Autodesk Inventor part; units mm, degrees
ref_plane "YZ Plane" through (0, 0, 0) normal (1, 0, 0) x (0, 1, 0)
ref_plane "XZ Plane" through (0, 0, 0) normal (0, 1, 0) x (-1, 0, 0)
ref_plane "XY Plane" through (0, 0, 0) normal (0, 0, 1) x (1, 0, 0)
sketch "Sketch5" plane through (0, 0, 0) normal (0, 0, 1) x (1, 0, 0)
  line L0 (27.5, -18) -> (0, -18)
  line L1 (0, -18) -> (0, 0)
  line L2 (27.5, -1.0645) -> (27.5, -18)
  line L3 (1.6866, 0) -> (2.5215, 2.0553)
  line L4 (2.5215, 2.0553) -> (3.0145, 0)
  line L5 (3.0145, 0) -> (3.8493, 2.0553)
  line L6 (3.8493, 2.0553) -> (4.3423, 0)
  line L7 (4.3423, 0) -> (5.1772, 2.0553)
  line L8 (5.1772, 2.0553) -> (5.6702, 0)
  line L9 (5.6702, 0) -> (6.505, 2.0553)
  line L10 (6.505, 2.0553) -> (6.998, 0)
  line L11 (6.998, 0) -> (7.8329, 2.0553)
  line L12 (7.8329, 2.0553) -> (8.4844, 0)
  line L13 (8.4844, 0) -> (9.3192, 2.0553)
  line L14 (9.3192, 2.0553) -> (9.9707, 0)
  line L15 (9.9707, 0) -> (10.8056, 2.0553)
  line L16 (10.8056, 2.0553) -> (11.4571, 0)
  line L17 (11.4571, 0) -> (12.292, 2.0553)
  line L18 (12.292, 2.0553) -> (12.9435, 0)
  line L19 (12.9435, 0) -> (13.7783, 2.0553)
  line L20 (13.7783, 2.0553) -> (14.4298, 0)
  line L21 (14.4298, 0) -> (15.4488, 2.0563)
  line L22 (15.4488, 2.0563) -> (16.0375, 0.0047)
  line L23 (16.0375, 0.0047) -> (16.8992, 2.0553)
  line L24 (16.8992, 2.0553) -> (17.489, 0)
  line L25 (0, 0) -> (1.6866, 0)
  line L26 (0, 0) -> (1.6866, 0)
  line L27 (17.489, 0) -> (18.3372, 2.0553)
  line L28 (18.3372, 2.0553) -> (18.989, -0.0011)
  line L29 (27.5, -0.0004) -> (27.5, -1.0645)
  line L30 (18.989, -0.0011) -> (19.8773, 2.0553)
  line L31 (19.8773, 2.0553) -> (20.4405, -0.0004)
  line L32 (15.4483, 2.0553) -> (15.4491, 2.0553)
  line L33 (18.9887, 0) -> (18.9895, 0)
  line L34 (20.4405, -0.0004) -> (27.5, -0.0004)
  point P0 (20.4491, -0.0317)
  dimension "d97" = 18
  dimension "d106" = 27.5
extrude "Extrusion2" add sketch "Sketch5" along normal blind 15
fillet "Fillet2" radius 15 1 edges at (0, -18, 7.5)
fillet "Rundung3" radius 5 1 edges at (0, 0, 7.5)
equation "\"l1\" = 8"
properties part number "Maria_Greifer_3D-Druck"
For this review, take the finished solid that the model builds, in its own axes (mm). Round coordinates to 2 decimals unless told otherwise and drop trailing zeros. Write each loop counter-clockwise with the first axis right and the second up, starting at its lowest first coordinate (ties: lowest second). Pieces come first, ordered by that corner, then holes. Notation, with made-up numbers: M 86.5,62 L 98.5,62 A33 ccw 98.5,98 Z; hole C 11.25,47.5 d1. An arc over 180 degrees is marked long. Write item = value, one per line. Start each with the question number.
(1) We need section C-C (y = -9.5). Give the boundary of the cut face in (x, z), then the cut area to 3 significant figures.
(2) For line 1 along Y through (x, z) = (21.25, 3.25); line 2 along X through (y, z) = (-9.5, 1); line 3 along X through (y, z) = (-12, 14), list the stretches that pass through material, from the lowest coordinate up.
(3) Clearance check with flat-ended pins moving along their axes: pin 1 Ø1 at (y, z) = (-0.5, 4.5) entering from -X; pin 2 Ø1.5 at (x, z) = (15, 12) entering from +Y; pin 3 Ø2 at (x, z) = (24.5, 5) entering from +Y. State where each tip first meets the part, or that it passes through.
(4) We need section B-B (x = 22.25). Give the boundary of the cut face in (y, z).
Results found:
q1.outline = M 1.48,0 L 27.5,0 L 27.5,15 L 1.48,15 Z
q1.area = 390 mm²
q2.line_1 = -18 to 0
q2.line_2 = 1.48 to 27.5
q2.line_3 = 3 to 27.5
q3.pin_1 = 0.83
q3.pin_2 = 2.06
q3.pin_3 = 0
q4.outline = M -18,0 L 0,0 L 0,15 L -18,15 Z
